Design review of the part shown in the three views and the two pictorial views. Dimensions are in mm from the part's minimum x, y and z. Coordinates: 2 decimals unless noted, no trailing zeros. Loops run counter-clockwise (first coordinate to the right, second up) from the corner with the lowest first, then second, coordinate; pieces in that order, holes last.
Q1. Draft analysis for pull direction X (two halves, no side actions). For the marked faces 1, 2, 3 and 4, state which applies: released by +X, released by -X, zero draft, split by the parting line, or undercut.
Q2. Add section C-C on z = 2.25. Give the boundary of the cut face in (x, y) (1 decimal).
Q3. Add section B-B on z = 4.75. Give the boundary of the cut face in (x, y) (1 decimal).
Q4. Wall thickness on probe 1 along Y at (x, z) = (28, 9); probe 2 along X at (y, z) = (3.5, 2.75) (1 decimal); probe 3 along X at (y, z) = (1.25, 7) (1 decimal): over which ranges is each line inside the solid? List them lowest first.
Q5. Add section A-A on y = 3.5. Give the boundary of the cut face in (x, z).
Q6. For P1, Ø3, axis at x = 19, y = 1, coming from the +Z side; P2, Ø1.8, axis at x = 38.5, y = 3, coming from the +Z side; P3, Ø3, axis at x = 2, y = 2.5, coming from the +Z side, all flat-tipped, find the tip position at first contact; note any pin that passes through.
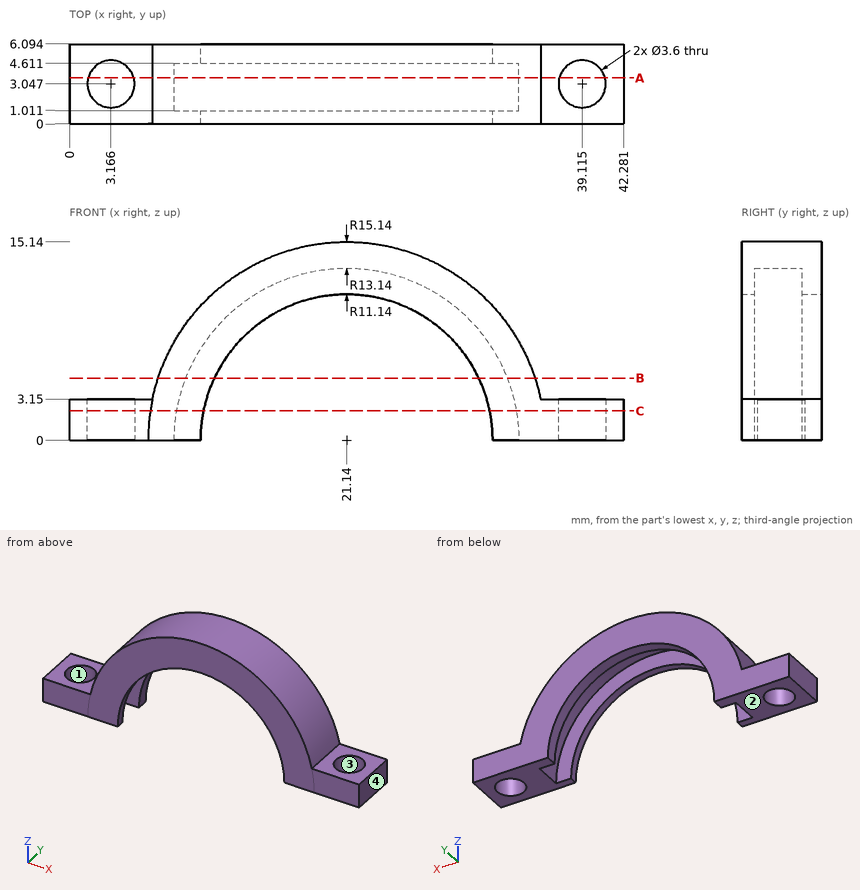
Entries:
1. face 1: undercut
1. face 2: zero draft
1. face 3: undercut
1. face 4: released by +X
2. outline: (0, 0) - (10.2, 0) - (10.2, 1) - (8.2, 1) - (8.2, 4.6) - (10.2, 4.6) - (10.2, 6.1) - (0, 6.1) - close; (32.1, 0) - (42.3, 0) - (42.3, 6.1) - (32.1, 6.1) - (32.1, 4.6) - (34.1, 4.6) - (34.1, 1) - (32.1, 1) - close; hole circle Ø3.6 at (3.2, 3); hole circle Ø3.6 at (39.1, 3)
3. outline: (6.8, 0) - (11.1, 0) - (11.1, 1) - (8.9, 1) - (8.9, 4.6) - (11.1, 4.6) - (11.1, 6.1) - (6.8, 6.1) - close; (31.2, 0) - (35.5, 0) - (35.5, 6.1) - (31.2, 6.1) - (31.2, 4.6) - (33.4, 4.6) - (33.4, 1) - (31.2, 1) - close
4. probe 1: y = 0 to 1.01, 4.61 to 6.09
4. probe 2: x = 0 to 1.4, 4.9 to 8.3, 34 to 37.4, 40.9 to 42.3
4. probe 3: x = 7.7 to 10, 32.3 to 34.6
5. outline: (0, 0) - (1.42, 0) - (1.42, 3.15) - (0, 3.15) - close; (4.91, 0) - (8, 0) arc R13.14 cw to (34.28, 0) - (37.37, 0) - (37.37, 3.15) - (35.95, 3.15) arc R15.14 ccw to (6.33, 3.15) - (4.91, 3.15) - close; (40.86, 0) - (42.28, 0) - (42.28, 3.15) - (40.86, 3.15) - close
6. P1: stops at z = 15.13
6. P2: passes through
6. P3: stops at z = 3.15
